from build123d import *

# Parameters (mm, degrees)
BOSS_EXTRUDE1_START = -152.4
SKETCH1_W           = 50.8
SKETCH1_H           = 6.35
BOSS_EXTRUDE1_DEPTH = 304.8
BOSS_EXTRUDE2_START = -12.7
BOSS_EXTRUDE2_DEPTH = 25.4
SKETCH2_R           = 1.651
CUT_EXTRUDE2_DEPTH  = 25.4
SKETCH3_R           = 1.9304
CUT_EXTRUDE4_DEPTH  = 25.4


with BuildPart() as part:
    # Sketch1 → Boss-Extrude1 (new body)
    with BuildSketch(Plane.XY.offset(BOSS_EXTRUDE1_START)):
        with Locations((25.4, -3.175)):
            Rectangle(SKETCH1_W, SKETCH1_H)
    extrude(amount=BOSS_EXTRUDE1_DEPTH)

    # Sketch1<7> → Boss-Extrude2 (add)
    with BuildSketch(Plane.XY.offset(BOSS_EXTRUDE2_START)):
        with BuildLine():
            ThreePointArc((50.8, -6.35), (53.483625962, -5.755054448), (55.664382214, -4.081701322))
            Line((55.664382214, -4.081701322), (104.644798072, 54.290885244))
            Line((104.644798072, 54.290885244), (99.780415858, 58.372586566))
            Line((99.780415858, 58.372586566), (50.8, 0))
            Line((50.8, 0), (50.8, -6.35))
        make_face()
    extrude(amount=BOSS_EXTRUDE2_DEPTH)

    # Sketch2 → Cut-Extrude2 (cut)
    with BuildSketch(Plane(origin=(0, 0, 0), x_dir=(1, 0, 0), z_dir=(0, 1, 0))):
        with Locations(Location((19.05, -139.7, 0), (0, 0, 270))):
            Circle(SKETCH2_R)
        with Locations(Location((31.75, -139.7, 0), (0, 0, 270))):
            Circle(SKETCH2_R)
        with Locations(Location((31.75, 139.7, 0), (0, 0, 270))):
            Circle(SKETCH2_R)
        with Locations(Location((19.05, 139.7, 0), (0, 0, 270))):
            Circle(SKETCH2_R)
    extrude(amount=-CUT_EXTRUDE2_DEPTH, mode=Mode.SUBTRACT)

    # Sketch3 → Cut-Extrude4 (cut)
    with BuildSketch(Plane(origin=(29.810663713, -25.014116927, 0), x_dir=(0.6427876096865373, 0.7660444431189797, 0), z_dir=(-0.7660444431189798, 0.6427876096865374, 0))):
        with Locations(Location((96.153610572, 0, 0), (0, 0, 180))):
            Circle(SKETCH3_R)
        with Locations(Location((58.053610572, 0, 0), (0, 0, 180))):
            Circle(SKETCH3_R)
    extrude(amount=-CUT_EXTRUDE4_DEPTH, mode=Mode.SUBTRACT)


solid = part.part
The model under review builds one solid part; all positions refer to its coordinate system, in mm. A direction names the side the tool comes from. Give positions to 0.01 mm unless a question says otherwise; leave off trailing zeros. Order: outer loops, then holes, each group sorted by start corner. A loop starts at its lowest first (then second) coordinate and runs counter-clockwise, first axis right, second up. Notation, with made-up numbers: M 21.25,-1.75 L 39.25,-1.75 A12 cw 39.25,16.25 Z; hole C 49.5,65 d4. An arc over 180 degrees is marked long. One line per question, with ' | ' between items. Start each with the question number.
1) For faces 1 (the face through (50.8, -3, -84)), 2 (the face through (25, -3, 152.4)), 3 (the face through (50.8, -3, 82)), list the 3-axis set-ups (+Z, -Z, +X, -X, +Y, -Y) from which the entire face can be reached by the end or side of a thin tool; tool diameter is ignored.
2) Consider section B-B, the plane x = 7. Give the boundary of the cut face in (y, z).
3) Consider section C-C, the plane y = 24.5. Give the boundary of the cut face in (x, z), then the cut area to 3 significant figures.
4) Consider section A-A, the plane z = -9.5. Give the boundary of the cut face in (x, y), then the cut area to 3 significant figures.
5) Clearance check with flat-ended pins moving along their axes: P1, Ø3, axis at y = -4, z = 54.5, coming from the +X side; P2, Ø12, axis at x = 34, z = 97, coming from the +Y side. State where each tip first meets the part, or that it passes through.
6) Wall thickness on L1, parallel to X at y = -2, z = 139.7; L2, parallel to Z at x = 19, y = -3; L3, parallel to Z at x = 31, y = -3: over which ranges is each line inside the solid? List them lowest first. Write a range as from..to.
7) Mouldability with a two-part tool opening along Z and no side actions: class faces 4 (the face through (0, -3, -2)), 5 (the face through (25, -3, -152.4)), 6 (the face through (95.255, 48.109, 0.085)) as pulls with the +Z half, pulls with the -Z half, needs draft (parallel to the pull), parting line crosses it, or undercut.
Found:
1) face 1: -Z, +X, +Y, -Y | face 2: +Z, +X, -X, +Y, -Y | face 3: +Z, +X, +Y, -Y
2) outline: M -6.35,-152.4 L 0,-152.4 L 0,152.4 L -6.35,152.4 Z
3) outline: M 71.36,-12.7 L 79.65,-12.7 L 79.65,12.7 L 71.36,12.7 Z | area: 211 mm²
4) outline: M 0,-6.35 L 50.8,-6.35 A6.35 ccw 55.66,-4.08 L 104.64,54.29 L 99.78,58.37 L 50.8,0 L 0,0 Z | area: 824 mm²
5) P1: stops at x = 50.8 | P2: stops at y = 0
6) L1: x = 0..17.4, 20.7..30.1, 33.4..50.8 | L2: z = -152.4..-141.35, -138.05..138.05, 141.35..152.4 | L3: z = -152.4..-141.17, -138.23..138.23, 141.17..152.4
7) face 4: needs draft | face 5: pulls with the -Z half | face 6: undercut
